Source: three-view drawing plus pictorial views. Frame: mm from the lowest corner of the part. A direction names the side the tool comes from. Round coordinates to 2 decimals unless told otherwise and drop trailing zeros. Write each loop counter-clockwise with the first axis right and the second up, starting at its lowest first coordinate (ties: lowest second). Pieces come first, ordered by that corner, then holes. Notation, with made-up numbers: M 22,4 L 68,4 A17 cw 68,16 Z; hole C 34.5,29.5 d2. An arc over 180 degrees is marked long. Put each result on its own line as item: value. Start each with the question number.
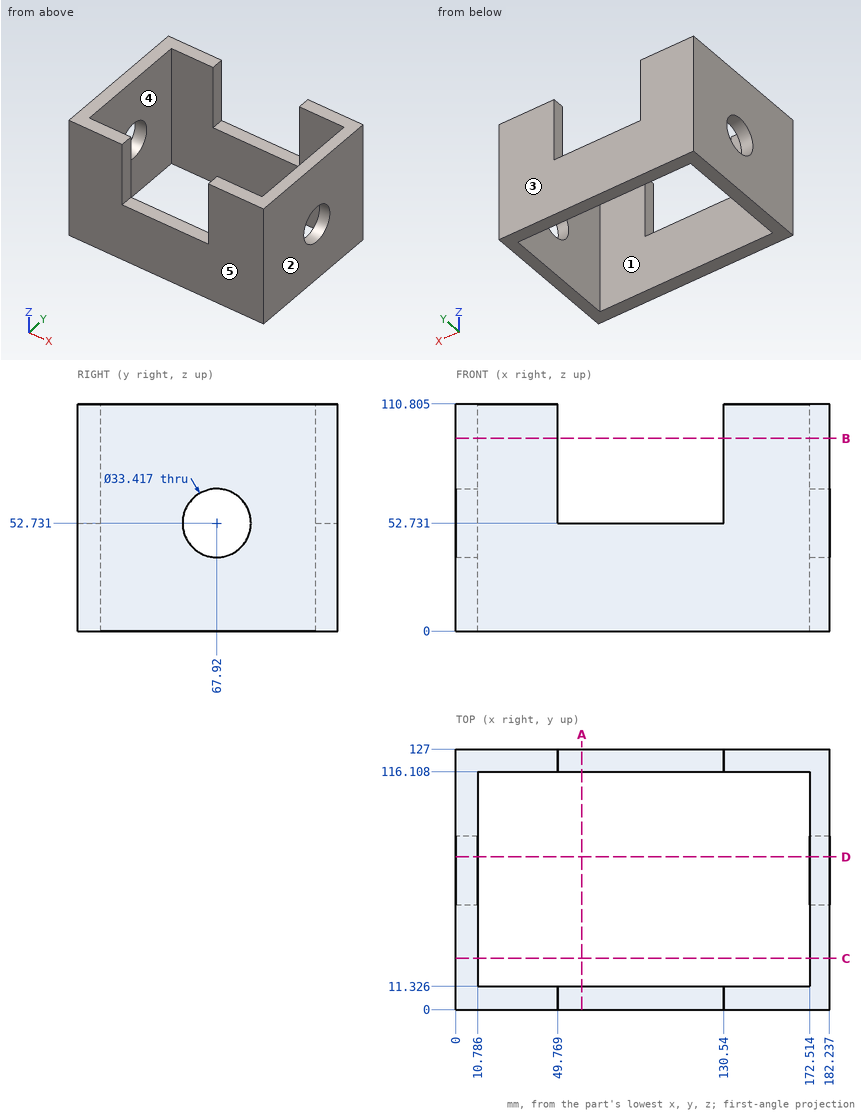
(1) Section query C-C (y = 25). Return loops of the section in (x, z) (1 decimal), and give its area (3 significant figures).
(2) Access query for the marked faces 4 and 5. Directions: +Z, -Z, +X, -X, +Y, -Y. A direction counts if a zero-diameter tool reaches every point of the face in a straight line with its end or side. Return the directions, or none.
(3) Section query A-A (x = 61.5). Return loops of the section in (y, z) (1 decimal).
(4) Section query D-D (y = 74.5). Return loops of the section in (x, z) (1 decimal), and give its area (3 significant figures).
(5) Ray query, line 1 along Y through (x, z) = (90.5, 18.5) (1 decimal); line 2 along X through (y, z) = (70, 16.5) (1 decimal); line 3 along Y through (x, z) = (173.5, 62). Return the intervals inside material, ascending.
(6) Pull-direction query (X, two-part tool) for the marked faces 1, 2 and 3; classes: +X half, -X half, draft (parallel to the pull), parting line (faces both ways), or undercut.
(7) Section query B-B (z = 94). Return loops of the section in (x, y) (1 decimal).
(8) Contact query for a flat-ended pin moving along its axis: P1, Ø3.5, axis at x = 88, y = 124, coming from the +Z side. Output: stop coordinate, or through.
Entries:
1. outline: M 0,0 L 10.8,0 L 10.8,110.8 L 0,110.8 Z; M 172.5,0 L 182.2,0 L 182.2,110.8 L 172.5,110.8 Z
1. area: 2,270 mm2
2. face 4: +Z, -Z
2. face 5: +Z, -Z, +X, -X, -Y
3. outline: M 0,0 L 11.3,0 L 11.3,52.7 L 0,52.7 Z; M 116.1,0 L 127,0 L 127,52.7 L 116.1,52.7 Z
4. outline: M 0,0 L 10.8,0 L 10.8,37.4 L 0,37.4 Z; M 0,68.1 L 10.8,68.1 L 10.8,110.8 L 0,110.8 Z; M 172.5,0 L 182.2,0 L 182.2,37.4 L 172.5,37.4 Z; M 172.5,68.1 L 182.2,68.1 L 182.2,110.8 L 172.5,110.8 Z
4. area: 1,640 mm2
5. line 1: 0 to 11.3, 116.1 to 127
5. line 2: 0 to 10.8, 172.5 to 182.2
5. line 3: 0 to 54.02, 81.82 to 127
6. face 1: undercut
6. face 2: +X half
6. face 3: draft
7. outline: M 0,0 L 49.8,0 L 49.8,11.3 L 10.8,11.3 L 10.8,116.1 L 49.8,116.1 L 49.8,127 L 0,127 Z; M 130.5,0 L 182.2,0 L 182.2,127 L 130.5,127 L 130.5,116.1 L 172.5,116.1 L 172.5,11.3 L 130.5,11.3 Z
8. P1: z = 52.73
